Could you check a few things on this drawing? It's one solid part, dimensions in mm from its lowest x, y, z. Give positions to 0.01 mm unless a question says otherwise; leave off trailing zeros. Loops run counter-clockwise (first coordinate to the right, second up) from the corner with the lowest first, then second, coordinate; pieces in that order, holes last. Notation, with made-up numbers: M 79,83.25 L 111,83.25 A18 ccw 111,112.25 Z; hole C 27,53.5 d7. An arc over 180 degrees is marked long. Write each question's results on one line, items separated by ' | '. Start each with the question number.
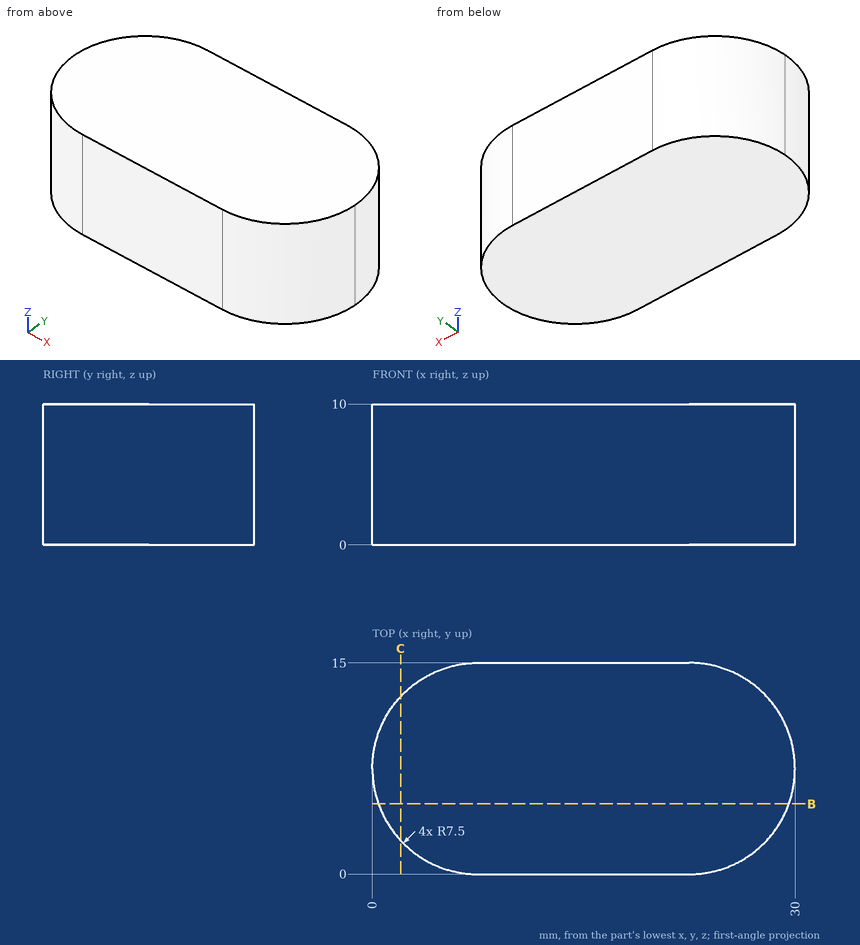
1) I'm going to push flat-ended pins straight in: P1, Ø4, axis at y = 11.5, z = 1.5, coming from the -X side; P2, Ø2, axis at y = 5, z = 2.5, coming from the +X side. Where does each tip first touch, or does it pass through?
2) If we section it at C-C on x = 2: Write out the boundary of the cut face in (y, z).
3) If we section it at B-B on y = 5: Write out the boundary of the cut face in (x, z).
4) Please list where these lines run through material, in increasing order: line 1 (X direction, y = 2.5, z = 0.5); line 2 (X direction, y = 11.25, z = 7.75) (1 decimal); line 3 (Y direction, x = 26.5, z = 4.5). Write a range as from..to.
Calculated:
1) P1: stops at x = 0.27 | P2: stops at x = 29.85
2) outline: M 2.4,0 L 12.6,0 L 12.6,10 L 2.4,10 Z
3) outline: M 0.43,0 L 29.57,0 L 29.57,10 L 0.43,10 Z
4) line 1: x = 1.91..28.09 | line 2: x = 1..29 | line 3: y = 1.16..13.84
